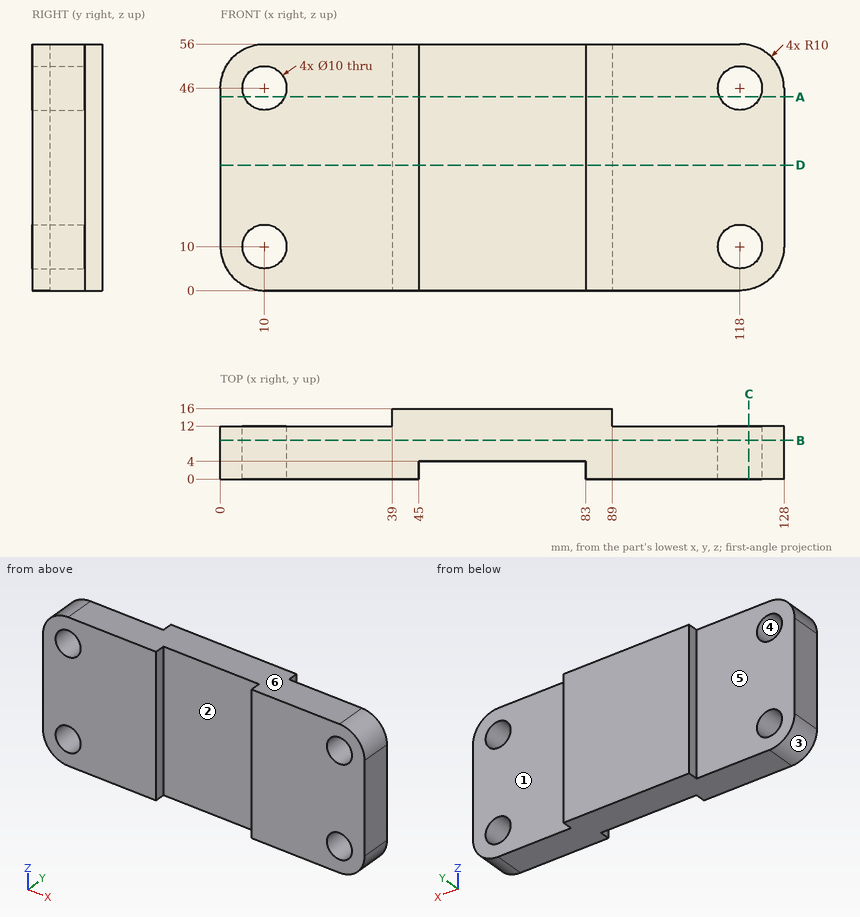
Geometry: see drawing. Coordinates: mm, zero at the bounding-box minimum. A direction names the side the tool comes from. Round coordinates to 2 decimals unless told otherwise and drop trailing zeros. Order: outer loops, then holes, each group sorted by start corner. A loop starts at its lowest first (then second) coordinate and runs counter-clockwise, first axis right, second up. Notation, with made-up numbers: (-37, 2.25) - (7, 2.25) arc R22 cw to (7, 36.25) - close; hole circle Ø8 at (75, 23). An arc over 180 degrees is marked (long way). Use a Markdown table: item, result. Add a question column.
1. Set-up query: the marked faces 1, 2 and 3. Return all of +Z, -Z, +X, -X, +Y, -Y with unobstructed straight access to the full face (end or side cutting, diameter ignored); none if empty.
2. Line query: probe 1 along X at (y, z) = (6.5, 46); probe 2 along Z at (x, y) = (118, 3.5); probe 3 along X at (y, z) = (8, 42). Output: solid intervals per line, ascending.
3. Mould query, pull axis Z, two halves, no side actions, for the marked faces 4, 5 and 6. Classes: +Z half, -Z half, draft (parallel to the pull), parting line (faces both ways), or undercut.
4. Section query A-A (z = 44). Return the cut outline in (x, y), then the cut area to 3 significant figures.
5. Section query D-D (z = 28.5). Return the cut outline in (x, y).
6. Section query C-C (x = 120). Return the cut outline in (y, z), then the cut area to 3 significant figures.
7. First-contact query: pin 1 (16 mm diameter, centred on x = 10, z = 10, fed in from +Y); pin 2 (11.5 mm diameter, centred on x = 70, z = 16.5, fed in from -Y); pin 3 (4.5 mm diameter, centred on y = 14.5, z = 41.5, fed in from -X). Flat tips, straight axial feed; report the tip coordinate or a pass-through.
8. Section query B-B (y = 8.75). Return the cut outline in (x, z), then the cut area to 3 significant figures.
Derived:
| question | item | result |
|---|---|---|
| 1 | face 1 | +Z, -Z, +X, +Y |
| 1 | face 2 | +Z, -Z, -Y |
| 1 | face 3 | -Z, -X, +Y, -Y |
| 2 | probe 1 | 0 to 5, 15 to 113, 123 to 128 |
| 2 | probe 2 | 0 to 5, 15 to 41, 51 to 56 |
| 2 | probe 3 | 0 to 7, 13 to 115, 121 to 128 |
| 3 | face 4 | undercut |
| 3 | face 5 | draft |
| 3 | face 6 | +Z half |
| 4 | outline | (0, 0) - (5.42, 0) - (5.42, 12) - (0, 12) - close; (14.58, 0) - (45, 0) - (45, 4) - (83, 4) - (83, 0) - (113.42, 0) - (113.42, 12) - (89, 12) - (89, 16) - (39, 16) - (39, 12) - (14.58, 12) - close; (122.58, 0) - (128, 0) - (128, 12) - (122.58, 12) - close |
| 4 | area | 1,360 mm2 |
| 5 | outline | (0, 0) - (45, 0) - (45, 4) - (83, 4) - (83, 0) - (128, 0) - (128, 12) - (89, 12) - (89, 16) - (39, 16) - (39, 12) - (0, 12) - close |
| 6 | outline | (0, 0.2) - (12, 0.2) - (12, 5.42) - (0, 5.42) - close; (0, 14.58) - (12, 14.58) - (12, 41.42) - (0, 41.42) - close; (0, 50.58) - (12, 50.58) - (12, 55.8) - (0, 55.8) - close |
| 6 | area | 447 mm2 |
| 7 | pin 1 | y = 12 |
| 7 | pin 2 | y = 4 |
| 7 | pin 3 | x = 39 |
| 8 | outline | (0, 10) arc R10 ccw to (10, 0) - (118, 0) arc R10 ccw to (128, 10) - (128, 46) arc R10 ccw to (118, 56) - (10, 56) arc R10 ccw to (0, 46) - close; hole circle Ø10 at (10, 10); hole circle Ø10 at (10, 46); hole circle Ø10 at (118, 10); hole circle Ø10 at (118, 46) |
| 8 | area | 6,770 mm2 |
